Input: part model. Units: mm. Frame: model coordinates. A direction names the side the tool comes from. Give positions to 0.01 mm unless a question says otherwise; leave off trailing zeros. Order: outer loops, then holes, each group sorted by start corner. A loop starts at its lowest first (then second) coordinate and runs counter-clockwise, first axis right, second up. Notation, with made-up numbers: M 62,3.5 L 100,3.5 A35 ccw 100,41.5 Z; hole C 80,-5.75 d6. An arc over 180 degrees is marked long. Use a Markdown table: item, result.
Autodesk Inventor part; units mm, degrees
ref_plane "Pracovní rovina1" through (20, 0, 0) normal (1, 0, 0) x (0, 1, 0)
ref_plane "Pracovní rovina2" through (-20, 0, 0) normal (1, 0, 0) x (0, 1, 0)
ref_plane "XZ Plane" through (0, 0, 0) normal (0, 1, 0) x (-1, 0, 0)
sketch "Náčrt1" plane through (0, 0, 0) normal (0, 0, 1) x (1, 0, 0)
  line L0 (-35, 35) -> (35, 35)
  line L1 (-35, 35) -> (0, -45)
  line L2 (0, -45) -> (35, 35)
  line L3 (0, 51) -> (0, -61)
  line L4 (-49, 0) -> (49, 0)
  line L5 (19.7098, 25) -> (-19.7098, 25)
  line L6 (-19.7098, 25) -> (0, -20.0511)
  line L7 (0, -20.0511) -> (19.7098, 25)
  point P0 (0, 0)
  dimension "d3" = 70
  dimension "d36" = 80
  dimension "d37" = 35
  dimension "d38" = 10
extrude "Vysunutí1" add sketch "Náčrt1" along normal mid plane 10 contours L0 L3 L5 L6 L4 L1 | L0 L2 L4 L7 L5 L3 | L4 L6 L3 L1 | L3 L7 L4 L2
fillet "Zaoblení1" radius 5 6 edges at (-35, 35, 0) (35, 35, 0) (0, -45, 0) (0, -20.0511, 0) (-19.7098, 25, 0) (19.7098, 25, 0)
ref_plane "Pracovní rovina1" through (20, 0, 0) normal (1, 0, 0) x (0, 1, 0)
ref_plane "Pracovní rovina2" through (-20, 0, 0) normal (1, 0, 0) x (0, 1, 0)
sketch "Náčrt3" plane through (20, 0, 0) normal (1, 0, 0) x (0, 1, 0)
  line L0 (45, -5) -> (30, -5)
  line L1 (30, -5) -> (30, 5)
  line L2 (30, 5) -> (45, 5)
  line L3 (45, 5) -> (45, -5)
  line L4 (35, 5) -> (35, -5)
  point P0 (0, 0)
  dimension "d18" = 15
  dimension "d19" = 10
  dimension "d20" = 10
sketch "Náčrt4" plane through (-20, 0, 0) normal (1, 0, 0) x (0, 1, 0)
  line L0 (35, -5) -> (27.9959, -5)
  line L1 (27.9959, -5) -> (27.9959, 5)
  line L2 (27.9959, 5) -> (35, 5)
  line L3 (35, 5) -> (35, -5)
  circle A0 centre (40, 0) radius 7.5
  point P0 (0, 0)
  point P1 (34.4098, -5)
  point P2 (34.4098, 5)
  dimension "d61" = 15
extrude "Vysunutí2" add sketch "Náčrt4" along normal mid plane 7
fillet "Zaoblení2" radius 3 2 edges at (-16.5, 35, 0) (-23.5, 35, 0)
ref_plane "Pracovní rovina7" through (23.5, 0, 0) normal (1, 0, 0) x (0, 0, -1)
sketch "Náčrt8" plane through (0, 0, 0) normal (1, 0, 0) x (0, 1, 0)
  line L0 (-54.0306, 0) -> (61.5051, 0)
  line L1 (0, 7) -> (0, -7)
  line L2 (27.9959, 5) -> (-34.5296, 5)
  arc A0 (38, -2.2361) -> (38, 2.2361) centre (40, 0) ccw
  line L3 (40, 0) -> (31.4495, 23.4923)
  line L4 (31.4495, 23.4923) -> (-33.0951, 0)
  line L5 (-33.0951, 0) -> (40, 0)
  line L6 (0, -7) -> (0, 7)
  line L7 (27.9959, -5) -> (-34.5296, -5)
  arc A1 (38, -2.2361) -> (38, 2.2361) centre (40, 0) ccw
  line L8 (40, 0) -> (31.4495, -23.4923)
  line L9 (31.4495, -23.4923) -> (-33.0951, 0)
  point P0 (0, 0)
  point P1 (-19.3577, 5)
  point P2 (0, 5)
  point P3 (0, -5)
  point P4 (-19.3577, -5)
  dimension "d47" = 25
  dimension "d48" = 20
  dimension "d49" = 90
  dimension "d50" = 0
ref_plane "Pracovní rovina6" through (10, 31.4495, -23.4923) normal (0, -0.342, -0.9397) x (-1, 0, 0)
sketch "Náčrt10" plane through (10, 31.4495, -23.4923) normal (0, -0.342, -0.9397) x (-1, 0, 0)
  line L0 (-47.61, -16.3764) -> (81.0156, -16.3764)
  line L1 (81.0156, -16.3764) -> (81.0156, -106.6518)
  line L2 (81.0156, -106.6518) -> (-47.61, -106.6518)
  line L3 (-47.61, -106.6518) -> (-47.61, -16.3764)
  point P0 (10, -37.5877)
extrude "Vysunutí8" cut sketch "Náčrt10" along normal blind 10
fillet "Zaoblení3" radius 15 2 edges at (-20, 34.4098, -5) (-20, 34.4098, 5)
mirror "Zrcadlit1" about plane through (0, 0, 0) normal (1, 0, 0) of "Vysunutí2", "Zaoblení2", "Zaoblení3"
sketch "Náčrt5" plane through (23.5, 0, 0) normal (1, 0, 0) x (0, 0, -1)
  line L0 (5, 35) -> (5, 45)
  line L1 (5, 45) -> (-5, 45)
  line L2 (-5, 45) -> (-5, 35)
  line L3 (5, 35) -> (-5, 35)
  point P0 (0, 0)
  point P1 (0, 40)
hole "Díra1" at (23.5, 40, 0) direction (1, 0, 0) diameter 6 end through all both
properties part number "trojúhleník_FF"
1) Cut plane C-C on z = -1.25. Return loops of the section in (x, y).
Response values:
| item | result |
|---|---|
| outline | M -31.94,28 L -6.71,-29.65 L 6.71,-29.65 L 31.94,28 A5 ccw 27.35,35 L 26.5,35 A3 cw 23.59,37.27 L 16.41,37.27 A3 cw 13.5,35 L -13.5,35 A3 cw -16.41,37.27 L -23.59,37.27 A3 cw -26.5,35 L -27.35,35 A5 ccw Z; M -23.5,42.73 L -16.5,42.73 L -16.5,47.4 L -23.5,47.4 Z; M 16.5,42.73 L 23.5,42.73 L 23.5,47.4 L 16.5,47.4 Z; hole M -16.65,18 L -4.58,-9.58 A5 ccw 4.58,-9.58 L 16.65,18 A5 ccw 12.06,25 L -12.06,25 A5 ccw Z |
2) Material intervals for line 1 (Z direction, x = -18.5, y = 40); line 2 (Y direction, x = 19.5, z = 0); line 3 (Z direction, x = -2, y = 29), sorted ascending. Write a range as from..to.
Response values:
| item | result |
|---|---|
| line 1 | z = -7.5..-3, 3..7.5 |
| line 2 | y = -0.43..37, 43..47.5 |
| line 3 | z = -5..5 |
3) Reachability of faces 1 (the face through (15.64, 35.9, -0.07)), 2 (the face through (14, 9, 5)), 3 (the face through (20, 37, 0)) from +Z, -Z, +X, -X, +Y, -Y: full face, straight path, thin tool, end or side. Return the list, or none.
Response values:
| item | result |
|---|---|
| face 1 | +Z, -Z, +Y |
| face 2 | +Z, -Y |
| face 3 | +X, -X |
4) First-contact query: pin 1 Ø4.5 at (y, z) = (39, -2) entering from -X; pin 2 Ø4 at (x, y) = (-2.5, -13) entering from +Z; pin 3 Ø6 at (y, z) = (36, -2.5) entering from +X. Flat tips, straight axial feed; report the tip coordinate or a pass-through.
Response values:
| item | result |
|---|---|
| pin 1 | stops at x = -23.77 |
| pin 2 | stops at z = 5 |
| pin 3 | stops at x = 31.35 |
5) Cut plane B-B on y = 40. Return loops of the section in (x, z).
Response values:
| item | result |
|---|---|
| outline | M -23.5,-7.5 L -16.5,-7.5 L -16.5,-3 L -23.5,-3 Z; M -23.5,3 L -16.5,3 L -16.5,7.5 L -23.5,7.5 Z; M 16.5,-7.5 L 23.5,-7.5 L 23.5,-3 L 16.5,-3 Z; M 16.5,3 L 23.5,3 L 23.5,7.5 L 16.5,7.5 Z |
6) Mould query, pull axis X, two halves, no side actions, for faces 4 (the face through (-23.5, 44, 0)), 5 (the face through (-0.081, -12.576, 0.07)), 6 (the face through (18.07, -3.7, -0.07)), 7 (the face through (19.951, 33.276, 5.434)). Classes: released by +X, released by -X, zero draft, split by the parting line, or undercut.
Response values:
| item | result |
|---|---|
| face 4 | released by -X |
| face 5 | undercut |
| face 6 | released by +X |
| face 7 | zero draft |
7) Cut plane D-D on x = 20. Return loops of the section in (y, z).
Response values:
| item | result |
|---|---|
| outline | M 0.71,-5 L 29.69,-5 A15 cw 36.56,-6.67 A7.5 ccw long 36.56,6.67 A15 cw 29.69,5 L 0.71,5 Z; hole C 40,0 d6 |
8) Cut plane A-A on x = 0. Return loops of the section in (y, z).
Response values:
| item | result |
|---|---|
| outline | M -37.53,1.61 L -19.35,-5 L -12.58,-5 L -12.58,5 L -37.53,5 Z; M 25,-5 L 35,-5 L 35,5 L 25,5 Z |
